from build123d import *

# Parameters (mm, degrees)
CROQUIS1_W              = 50.3
CROQUIS1_H              = 10.7
SALIENTE_EXTRUIR1_DEPTH = 15.7
CORTAR_EXTRUIR1_REACH   = 55.769
CROQUIS2_W              = 10
CROQUIS2_H              = 10.7
CORTAR_EXTRUIR2_REACH   = 55.769
CROQUIS3_W              = 20.3
CROQUIS3_H              = 9.2
CORTAR_EXTRUIR3_REACH   = 46.554
CROQUIS4_W              = 1.5
CROQUIS4_H              = 4.7
CORTAR_EXTRUIR5_REACH   = 54.527
CROQUIS6_R              = 3
CORTAR_EXTRUIR6_REACH   = 54.421
CROQUIS7_R              = 1.5
CORTAR_EXTRUIR7_DEPTH   = 3
SALIENTE_EXTRUIR2_DEPTH = 5
CROQUIS11_W             = 5
CROQUIS11_H             = 4.7
SALIENTE_EXTRUIR3_DEPTH = 2.3
CROQUIS12_W             = 10
CROQUIS12_H             = 5
SALIENTE_EXTRUIR5_DEPTH = 3
CROQUIS13_W             = 15
CROQUIS13_H             = 5
SALIENTE_EXTRUIR6_DEPTH = 5
CROQUIS14_W             = 5
CROQUIS14_H             = 8
SALIENTE_EXTRUIR7_DEPTH = 10.3


with BuildPart() as part:
    # Croquis1 → Saliente-Extruir1 (new body)
    with BuildSketch(Plane(origin=(0, 0, 0), x_dir=(1, 0, 0), z_dir=(0, 1, 0))):
        with Locations((-25.15, -5.35)):
            Rectangle(CROQUIS1_W, CROQUIS1_H)
    extrude(amount=SALIENTE_EXTRUIR1_DEPTH)

    # Croquis2 → Cortar-Extruir1 (cut, up to next)
    with BuildSketch(Plane.XY.offset(10.7), mode=Mode.PRIVATE) as cortar_extruir1_sk1:
        with Locations((-45.3, 10.35)):
            Rectangle(CROQUIS2_W, CROQUIS2_H)
    cortar_extruir1_tool1 = extrude(cortar_extruir1_sk1.sketch, amount=-CORTAR_EXTRUIR1_REACH, mode=Mode.PRIVATE) & part.part
    # Croquis2 → Cortar-Extruir1 (cut, up to next)
    with BuildSketch(Plane.XY.offset(10.7), mode=Mode.PRIVATE) as cortar_extruir1_sk2:
        with BuildLine():
            Line((-35.3, 5.532906309), (-15, 5.532906309))
            Line((-15, 5.532906309), (-15, 12.532906309))
            ThreePointArc((-15, 12.532906309), (-15.292893219, 13.240013091), (-16, 13.532906309))
            Line((-16, 13.532906309), (-34.3, 13.532906309))
            ThreePointArc((-34.3, 13.532906309), (-35.007106781, 13.240013091), (-35.3, 12.532906309))
            Line((-35.3, 12.532906309), (-35.3, 5.532906309))
        make_face()
    cortar_extruir1_tool2 = extrude(cortar_extruir1_sk2.sketch, amount=-CORTAR_EXTRUIR1_REACH, mode=Mode.PRIVATE) & part.part
    # Croquis2 → Cortar-Extruir1 (cut, up to next)
    with BuildSketch(Plane.XY.offset(10.7), mode=Mode.PRIVATE) as cortar_extruir1_sk3:
        with Locations((-5, 10.35)):
            Rectangle(CROQUIS2_W, CROQUIS2_H)
    cortar_extruir1_tool3 = extrude(cortar_extruir1_sk3.sketch, amount=-CORTAR_EXTRUIR1_REACH, mode=Mode.PRIVATE) & part.part
    add(cortar_extruir1_tool1.solids().sort_by_distance((-45.3, 10.35, 10.7))[0], mode=Mode.SUBTRACT)
    add(cortar_extruir1_tool2.solids().sort_by_distance((-25.15, 9.522899, 10.7))[0], mode=Mode.SUBTRACT)
    add(cortar_extruir1_tool3.solids().sort_by_distance((-5, 10.35, 10.7))[0], mode=Mode.SUBTRACT)

    # Croquis3 → Cortar-Extruir2 (cut, up to next)
    with BuildSketch(Plane(origin=(0, 15.7, 0), x_dir=(1, 0, 0), z_dir=(0, 1, 0)), mode=Mode.PRIVATE) as cortar_extruir2_sk1:
        with Locations((-25.15, -4.6)):
            Rectangle(CROQUIS3_W, CROQUIS3_H)
    cortar_extruir2_tool1 = extrude(cortar_extruir2_sk1.sketch, amount=-CORTAR_EXTRUIR2_REACH, mode=Mode.PRIVATE) & part.part
    add(cortar_extruir2_tool1.solids().sort_by_distance((-25.15, 15.7, 4.6))[0], mode=Mode.SUBTRACT)

    # Croquis4 → Cortar-Extruir3 (cut, up to next)
    with BuildSketch(Plane.ZY.offset(40.3), mode=Mode.PRIVATE) as cortar_extruir3_sk1:
        with Locations((0.75, 13.35)):
            Rectangle(CROQUIS4_W, CROQUIS4_H)
    cortar_extruir3_tool1 = extrude(cortar_extruir3_sk1.sketch, amount=-CORTAR_EXTRUIR3_REACH, mode=Mode.PRIVATE) & part.part
    add(cortar_extruir3_tool1.solids().sort_by_distance((-40.3, 13.35, 0.75))[0], mode=Mode.SUBTRACT)

    # Croquis6 → Cortar-Extruir5 (cut, up to next)
    with BuildSketch(Plane(origin=(0, 5, 0), x_dir=(1, 0, 0), z_dir=(0, 1, 0)), mode=Mode.PRIVATE) as cortar_extruir5_sk1:
        with Locations(Location((-45.3, -4.941101113, 0), (0, 0, 270))):
            Circle(CROQUIS6_R)
    cortar_extruir5_tool1 = extrude(cortar_extruir5_sk1.sketch, amount=-CORTAR_EXTRUIR5_REACH, mode=Mode.PRIVATE) & part.part
    # Croquis6 → Cortar-Extruir5 (cut, up to next)
    with BuildSketch(Plane(origin=(0, 5, 0), x_dir=(1, 0, 0), z_dir=(0, 1, 0)), mode=Mode.PRIVATE) as cortar_extruir5_sk2:
        with Locations(Location((-5, -4.941101113, 0), (0, 0, 90))):
            Circle(CROQUIS6_R)
    cortar_extruir5_tool2 = extrude(cortar_extruir5_sk2.sketch, amount=-CORTAR_EXTRUIR5_REACH, mode=Mode.PRIVATE) & part.part
    add(cortar_extruir5_tool1.solids().sort_by_distance((-45.3, 5, 4.941101))[0], mode=Mode.SUBTRACT)
    add(cortar_extruir5_tool2.solids().sort_by_distance((-5, 5, 4.941101))[0], mode=Mode.SUBTRACT)

    # Croquis7 → Cortar-Extruir6 (cut, up to next)
    with BuildSketch(Plane(origin=(0, 5.532906309, 0), x_dir=(1, 0, 0), z_dir=(0, 1, 0)), mode=Mode.PRIVATE) as cortar_extruir6_sk1:
        with Locations(Location((-30.3, -2.6, 0), (0, 0, 270))):
            Circle(CROQUIS7_R)
    cortar_extruir6_tool1 = extrude(cortar_extruir6_sk1.sketch, amount=-CORTAR_EXTRUIR6_REACH, mode=Mode.PRIVATE) & part.part
    # Croquis7 → Cortar-Extruir6 (cut, up to next)
    with BuildSketch(Plane(origin=(0, 5.532906309, 0), x_dir=(1, 0, 0), z_dir=(0, 1, 0)), mode=Mode.PRIVATE) as cortar_extruir6_sk2:
        with Locations(Location((-20, -2.6, 0), (0, 0, 270))):
            Circle(CROQUIS7_R)
    cortar_extruir6_tool2 = extrude(cortar_extruir6_sk2.sketch, amount=-CORTAR_EXTRUIR6_REACH, mode=Mode.PRIVATE) & part.part
    add(cortar_extruir6_tool1.solids().sort_by_distance((-30.3, 5.532906, 2.6))[0], mode=Mode.SUBTRACT)
    add(cortar_extruir6_tool2.solids().sort_by_distance((-20, 5.532906, 2.6))[0], mode=Mode.SUBTRACT)

    # Croquis8 → Cortar-Extruir7 (cut)
    with BuildSketch(Plane(origin=(0, 5, 0), x_dir=(1, 0, 0), z_dir=(0, 1, 0))):
        Polygon((-5, -0.1), (-9.54663337, -2.725), (-9.54663337, -7.975), (-5, -10.6), (-0.45336663, -7.975), (-0.45336663, -2.725), align=None)
        Polygon((-49.84663337, -2.725), (-45.3, -0.1), (-40.75336663, -2.725), (-40.75336663, -7.975), (-45.3, -10.6), (-49.84663337, -7.975), align=None)
    extrude(amount=-CORTAR_EXTRUIR7_DEPTH, mode=Mode.SUBTRACT)

    # Croquis9 → Saliente-Extruir2 (add)
    with BuildSketch(Plane(origin=(-35.3, 0, 0), x_dir=(0, 0, -1), z_dir=(1, 0, 0))):
        Polygon((-1.5, 15.7), (2.7, 15.7), (2.7, 11), (4.7, 11), (4.7, 20.7), (-5.753105751, 20.7), (-5.753105751, 15.7), align=None)
    extrude(amount=-SALIENTE_EXTRUIR2_DEPTH)

    # Croquis11 → Saliente-Extruir3 (add)
    with BuildSketch(Plane(origin=(0, 0, 0), x_dir=(-1, 0, 0), z_dir=(0, 0, -1))):
        with Locations((12.5, 13.35)):
            Rectangle(CROQUIS11_W, CROQUIS11_H)
    extrude(amount=SALIENTE_EXTRUIR3_DEPTH)

    # Croquis12 → Saliente-Extruir5 (add)
    with BuildSketch(Plane(origin=(0, 15.7, 0), x_dir=(1, 0, 0), z_dir=(0, 1, 0))):
        with Locations((-20, -0.2)):
            Rectangle(CROQUIS12_W, CROQUIS12_H)
    extrude(amount=-SALIENTE_EXTRUIR5_DEPTH)

    # Croquis13 → Saliente-Extruir6 (add)
    with BuildSketch(Plane(origin=(0, 15.7, 0), x_dir=(1, 0, 0), z_dir=(0, 1, 0))):
        with Locations((-17.5, -0.2)):
            Rectangle(CROQUIS13_W, CROQUIS13_H)
    extrude(amount=SALIENTE_EXTRUIR6_DEPTH)

    # Croquis14 → Saliente-Extruir7 (add)
    with BuildSketch(Plane.ZY.offset(25)):
        with Locations((0.2, 16.7)):
            Rectangle(CROQUIS14_W, CROQUIS14_H)
    extrude(amount=SALIENTE_EXTRUIR7_DEPTH)


solid = part.part
For this review, take the finished solid that the model builds, in its own axes (mm). A direction names the side the tool comes from. Coordinates: 2 decimals unless noted, no trailing zeros. Loops run counter-clockwise (first coordinate to the right, second up) from the corner with the lowest first, then second, coordinate; pieces in that order, holes last. Notation, with made-up numbers: (-14, 11) - (2, 11) arc R8 cw to (2, 22) - close; hole circle Ø9 at (43.25, 75). An arc over 180 degrees is marked (long way). Return JSON: item names as keys, results as strings.
Item 1: Take a section at D-D (z = 7). Give the boundary of the cut face in (x, y), then the cut area to 3 significant figures.
Determined:
{"outline": "(-50.3, 0) - (-47.48, 0) - (-47.48, 2) - (-49.85, 2) - (-49.85, 5) - (-50.3, 5) - close; (-43.12, 0) - (-7.18, 0) - (-7.18, 2) - (-9.55, 2) - (-9.55, 5) - (-10, 5) - (-10, 15.7) - (-15, 15.7) - (-15, 5.53) - (-35.3, 5.53) - (-35.3, 15.7) - (-40.3, 15.7) - (-40.3, 5) - (-40.75, 5) - (-40.75, 2) - (-43.12, 2) - close; (-2.82, 0) - (0, 0) - (0, 5) - (-0.45, 5) - (-0.45, 2) - (-2.82, 2) - close", "area": "297 mm2"}
Item 2: Insertion check: pin 1 (2 mm diameter, centred on y = 12, z = 0.5, fed in from +X); pin 2 (8 mm diameter, centred on x = -27, y = 14.5, fed in from -Z); pin 3 (2 mm diameter, centred on x = -36.5, z = -3.5, fed in from -Y); pin 4 (4 mm diameter, centred on x = -26.5, y = 10, fed in from -Z). Each pin has a flat end and moves straight along its axis. Give the tip position at first contact, or say it passes through.
Determined:
{"pin 1": "stops at x = -10", "pin 2": "stops at z = -2.3", "pin 3": "stops at y = 11", "pin 4": "passes through"}
Item 3: For faces 1 (the flat face through (-35.3, 14, 0)), 2 (the flat face through (-7, 5, 10)), 3 (the flat face through (-9.547, 4, 5)), 4 (the flat face through (-15, 11, 6)), list the 3-axis set-ups (+Z, -Z, +X, -X, +Y, -Y) from which the entire face can be reached by the end or side of a thin tool; tool diameter is ignored.
Determined:
{"face 1": "-X", "face 2": "+Z, -Z, +X, +Y", "face 3": "+Y", "face 4": "none"}
Item 4: Take a section at B-B (x = -30.3). Give the boundary of the cut face in (y, z).
Determined:
{"outline": "(0, 0) - (5.53, 0) - (5.53, 1.1) - (0, 1.1) - close; (0, 4.1) - (5.53, 4.1) - (5.53, 10.7) - (0, 10.7) - close; (12.7, -2.3) - (20.7, -2.3) - (20.7, 2.7) - (12.7, 2.7) - close; (13.53, 9.2) - (15.7, 9.2) - (15.7, 10.7) - (13.53, 10.7) - close"}
Item 5: Mouldability with a two-part tool opening along Z and no side actions: class faces 5 (the flat face through (-26, 4, 10.7)), 6 (the flat face through (-25, 5.533, 5)), 7 (the flat face through (-38, 13, -2.7)) as pulls with the +Z half, pulls with the -Z half, needs draft (parallel to the pull), parting line crosses it, or undercut.
Determined:
{"face 5": "pulls with the +Z half", "face 6": "needs draft", "face 7": "undercut"}
Item 6: Take a section at A-A (y = 7). Give the boundary of the cut face in (x, z).
Determined:
{"outline": "(-40.3, 0) - (-35.3, 0) - (-35.3, 10.7) - (-40.3, 10.7) - close; (-15, 0) - (-10, 0) - (-10, 10.7) - (-15, 10.7) - close"}
Item 7: Take a section at C-C (y = 1.5). Give the boundary of the cut face in (x, z), then the cut area to 3 significant figures.
Determined:
{"outline": "(-50.3, 0) - (0, 0) - (0, 10.7) - (-50.3, 10.7) - close; hole circle Ø6 at (-45.3, 4.94); hole circle Ø3 at (-30.3, 2.6); hole circle Ø3 at (-20, 2.6); hole circle Ø6 at (-5, 4.94)", "area": "468 mm2"}
Item 8: For line 1 (Y direction, x = -23, z = 9.75); line 2 (X direction, y = 10.25, z = 4.25); line 3 (X direction, y = 2.25, z = 4.25), list the stretches that pass through material, from the lowest coordinate up.
Determined:
{"line 1": "y = 0 to 5.53, 13.53 to 15.7", "line 2": "x = -40.3 to -35.3, -15 to -10", "line 3": "x = -50.3 to -49.85, -40.75 to -9.55, -0.45 to 0"}
